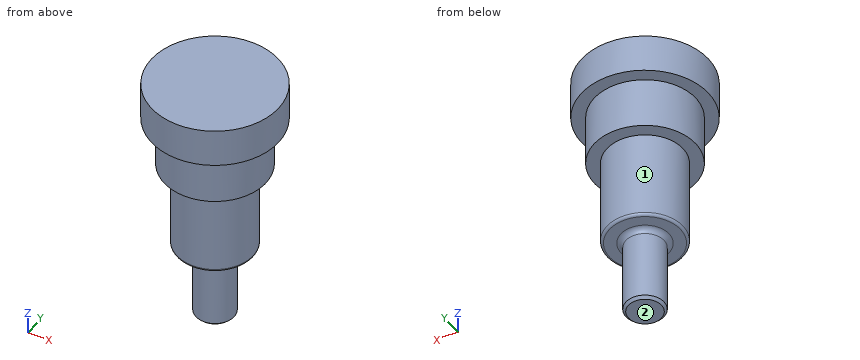
Autodesk Inventor part; units mm, degrees
ref_plane "YZ Plane" through (0, 0, 0) normal (1, 0, 0) x (0, 1, 0)
ref_plane "XZ Plane" through (0, 0, 0) normal (0, 1, 0) x (-1, 0, 0)
ref_plane "XY Plane" through (0, 0, 0) normal (0, 0, 1) x (1, 0, 0)
sketch "Sketch1" plane through (0, 0, 0) normal (1, 0, 0) x (0, 1, 0)
  line L0 (0, 0) -> (0, -100)
  line L1 (0, -100) -> (7.5, -100)
  line L2 (7.5, -100) -> (7.5, -70)
  line L3 (7.5, -70) -> (15, -70)
  line L4 (15, -70) -> (15, -35)
  line L5 (15, -35) -> (20, -35)
  line L6 (20, -35) -> (20, -15)
  line L7 (20, -15) -> (25, -15)
  line L8 (25, -15) -> (25, 0)
  line L9 (25, 0) -> (0, 0)
  dimension "d0" = 100
  dimension "d1" = 15
  dimension "d2" = 20
  dimension "d3" = 35
  dimension "d4" = 15
  dimension "d5" = 30
  dimension "d6" = 40
  dimension "d7" = 50
revolve "Revolution1" add sketch "Sketch1" angle 360 mid plane about axis through (0, 0, 0) along (0, 0, -1)
chamfer "Chamfer1" distance 1 angle 45 1 edges at (0, 7.5, -100)
fillet "Fillet1" radius 2 1 edges at (0, 7.5, -70)
fillet "Fillet2" radius 1 1 edges at (0, 15, -70)
thread "Thread1"
Verification items for the finished model (mm, model axes). Face numbers are marked on the shaded views. A direction names the side the tool comes from. Coordinates: 2 decimals unless noted, no trailing zeros. Loops run counter-clockwise (first coordinate to the right, second up) from the corner with the lowest first, then second, coordinate; pieces in that order, holes last. Notation, with made-up numbers: (27, -19.75) -> (55, -19.75) arc R12 ccw to (55, -5.75) -> close; hole circle Ø5 at (64, 20.25). An arc over 180 degrees is marked (long way). Answer in a Markdown table with one row per item. Add a question column.
1. Material ranges on probe 1 along Z at (x, y) = (18.5, 11); probe 2 along Z at (x, y) = (14, -10.5); probe 3 along X at (y, z) = (-13, -59), recorded low to high. Write a range as [from, to].
2. Section check C-C, the plane z = -24. Enter the section's corners in (x, y), then the cut area to 3 significant figures.
3. Depth check by flat-ended pin: P1, Ø10, axis at x = -11, z = -22.5, coming from the -Y side; P2, Ø6, axis at x = -5.5, z = -55.5, coming from the -Y side; P3, Ø5, axis at x = 9, z = -76.5, coming from the +Y side; P4, Ø4, axis at x = -3, y = -18, coming from the +Z side. Enter the tip coordinate at first touch or a pass-through.
4. Section check A-A, the plane y = 0. Enter the section's corners in (x, z), then the cut area to 3 significant figures.
5. Access from +Z, -Z, +X, -X, +Y, -Y to the whole of each face (thin tool, end or side, straight path). Record for the marked faces 1 and 2.
6. Section check D-D, the plane x = -17. Enter the section's corners in (y, z).
Derived:
| question | item | result |
|---|---|---|
| 1 | probe 1 | z = [-15, 0] |
| 1 | probe 2 | z = [-35, 0] |
| 1 | probe 3 | x = [-7.48, 7.48] |
| 2 | outline | circle Ø40 at (0, 0) |
| 2 | area | 1,260 mm² |
| 3 | P1 | stops at y = -19.08 |
| 3 | P2 | stops at y = -14.79 |
| 3 | P3 | stops at y = 3.74 |
| 3 | P4 | stops at z = 0 |
| 4 | outline | (-25, -15) -> (-20, -15) -> (-20, -35) -> (-15, -35) -> (-15, -69) arc R1 ccw to (-14, -70) -> (-9.5, -70) arc R2 cw to (-7.5, -72) -> (-7.5, -99) -> (-6.5, -100) -> (6.5, -100) -> (7.5, -99) -> (7.5, -72) arc R2 cw to (9.5, -70) -> (14, -70) arc R1 ccw to (15, -69) -> (15, -35) -> (20, -35) -> (20, -15) -> (25, -15) -> (25, 0) -> (-25, 0) -> close |
| 4 | area | 3,050 mm² |
| 5 | face 1 | -Z |
| 5 | face 2 | -Z, +X, -X, +Y, -Y |
| 6 | outline | (-18.33, -15) -> (-10.54, -15) -> (-10.54, -35) -> (10.54, -35) -> (10.54, -15) -> (18.33, -15) -> (18.33, 0) -> (-18.33, 0) -> close |
